from build123d import *

# Parameters (mm, degrees)
SKETCH1_W                    = 110
SKETCH1_H                    = 50
BASE_FLANGE1_DEPTH           = 6
CUT_EXTRUDE1_DEPTH           = 10
LPATTERN1_COUNT              = 2
LPATTERN1_PITCH              = 57
MIRROR1_COPY_1_DEPTH         = 10
EDGE_FLANGE1_STRIP_W         = 40
EDGE_FLANGE1_STRIP_H         = 6
EDGE_FLANGE1_STRIP_CUT_DEPTH = 50
EDGE_FLANGE1_DEPTH           = 50
EDGE_FLANGE2_STRIP_W         = 40
EDGE_FLANGE2_STRIP_H         = 6
EDGE_FLANGE2_STRIP_CUT_DEPTH = 50
EDGE_FLANGE2_DEPTH           = 50
SKETCH9_R                    = 4.5
CUT_EXTRUDE2_DEPTH           = 10


# Sheet-metal steps are written as plain solids
with BuildPart() as part:
    # Sketch1 → Base-Flange1 (new body)
    with BuildSketch(Plane(origin=(0, 0, 0), x_dir=(0, 0, -1), z_dir=(1, 0, 0))):
        Rectangle(SKETCH1_W, SKETCH1_H)
    extrude(amount=-BASE_FLANGE1_DEPTH)

    # Sketch5 → Cut-Extrude1 (cut)
    with BuildSketch(Plane.ZY.offset(6)):
        with BuildLine():
            Line((-30, 13), (-10, 13))
            ThreePointArc((-10, 13), (-7.5, 10.5), (-10, 8))
            Line((-10, 8), (-30, 8))
            ThreePointArc((-30, 8), (-32.5, 10.5), (-30, 13))
        make_face()
    cut_extrude1 = extrude(amount=-CUT_EXTRUDE1_DEPTH, mode=Mode.SUBTRACT)

    # LPattern1: Cut-Extrude1 ×2
    with Locations(*[(0, 0, i * LPATTERN1_PITCH) for i in range(1, LPATTERN1_COUNT)]):
        add(cut_extrude1, mode=Mode.SUBTRACT)

    # Mirror1: Cut-Extrude1 across plane
    add(cut_extrude1.mirror(Plane.ZX), mode=Mode.SUBTRACT)

    # Mirror1 copy 1 sketch → Mirror1 copy 1 (cut)
    with BuildSketch(Plane(origin=(-6, 0, 57), x_dir=(0, 0, 1), z_dir=(-1, 0, 0))):
        with BuildLine():
            Line((-30, -13), (-10, -13))
            ThreePointArc((-10, -13), (-7.5, -10.5), (-10, -8))
            Line((-10, -8), (-30, -8))
            ThreePointArc((-30, -8), (-32.5, -10.5), (-30, -13))
        make_face()
    extrude(amount=-MIRROR1_COPY_1_DEPTH, mode=Mode.SUBTRACT)

    # Edge-Flange1 strip (across the edge) → Edge-Flange1 strip cut (cut)
    with BuildSketch(Plane(origin=(0, -25, -55), x_dir=(0, 0, 1), z_dir=(0, 1, 0))):
        with Locations((-6, -3)):
            Rectangle(EDGE_FLANGE1_STRIP_W, EDGE_FLANGE1_STRIP_H)
    extrude(amount=EDGE_FLANGE1_STRIP_CUT_DEPTH, mode=Mode.SUBTRACT)

    # Edge-Flange1 section (across the edge) → Edge-Flange1 (add)
    with BuildSketch(Plane(origin=(0, -25, -55), x_dir=(0, 0, 1), z_dir=(0, 1, 0))):
        with BuildLine():
            Line((0, 8), (0, 67))
            Line((0, 67), (6, 67))
            Line((6, 67), (6, 8))
            ThreePointArc((6, 8), (8.343145751, 2.343145751), (14, 0))
            Line((14, 0), (14, -6))
            ThreePointArc((14, -6), (4.100505063, -1.899494937), (0, 8))
        make_face()
    extrude(amount=EDGE_FLANGE1_DEPTH)

    # Edge-Flange2 strip (across the edge) → Edge-Flange2 strip cut (cut)
    with BuildSketch(Plane(origin=(67, 25, -55), x_dir=(-1, 0, 0), z_dir=(0, -1, 0))):
        with Locations((-6, -3)):
            Rectangle(EDGE_FLANGE2_STRIP_W, EDGE_FLANGE2_STRIP_H)
    extrude(amount=EDGE_FLANGE2_STRIP_CUT_DEPTH, mode=Mode.SUBTRACT)

    # Edge-Flange2 section (across the edge) → Edge-Flange2 (add)
    with BuildSketch(Plane(origin=(67, 25, -55), x_dir=(-1, 0, 0), z_dir=(0, -1, 0))):
        with BuildLine():
            Line((0, 8), (0, 104))
            Line((0, 104), (6, 104))
            Line((6, 104), (6, 8))
            ThreePointArc((6, 8), (8.343145751, 2.343145751), (14, 0))
            Line((14, 0), (14, -6))
            ThreePointArc((14, -6), (4.100505063, -1.899494937), (0, 8))
        make_face()
    extrude(amount=EDGE_FLANGE2_DEPTH)

    # Sketch9 → Cut-Extrude2 (cut)
    with BuildSketch(Plane.ZY.offset(-61)):
        with Locations((-94, 0)):
            Circle(SKETCH9_R)
    extrude(amount=-CUT_EXTRUDE2_DEPTH, mode=Mode.SUBTRACT)

    # Mirror2: part across plane


with BuildPart() as part_1:
    add(part.part)
    add(part.part.mirror(Plane(origin=(67, 25, -159), x_dir=(1, 0, 0), z_dir=(0, 0, 1))))


solid = part_1.part
Model file for the job. Use its own axes, mm. A direction names the side the tool comes from. Give positions to 0.01 mm unless a question says otherwise; leave off trailing zeros. Order: outer loops, then holes, each group sorted by start corner. A loop starts at its lowest first (then second) coordinate and runs counter-clockwise, first axis right, second up. Notation, with made-up numbers: (-29.5, -2.75) - (-18.5, -2.75) arc R31 cw to (-18.5, 35.25) - close; hole circle Ø10 at (20.25, 11). An arc over 180 degrees is marked (long way). Return JSON: item names as keys, results as strings.
1) Cut at C-C, the plane z = -0.5. Give the cut face in (x, y), plus the area to 3 significant figures.
Geometry says:
{"outline": "(-6, -25) - (0, -25) - (0, 25) - (-6, 25) - close", "area": "300 mm²"}
2) Cut at B-B, the plane z = -94. Give the cut face in (x, y), plus the area to 3 significant figures.
Geometry says:
{"outline": "(61, -25) - (67, -25) - (67, -4.5) - (61, -4.5) - close; (61, 4.5) - (67, 4.5) - (67, 25) - (61, 25) - close", "area": "246 mm²"}
3) Cut at A-A, the plane x = 23.5. Give the cut face in (y, z), plus the area to 3 significant figures.
Geometry says:
{"outline": "(-25, -269) - (25, -269) - (25, -263) - (-25, -263) - close; (-25, -55) - (25, -55) - (25, -49) - (-25, -49) - close", "area": "600 mm²"}
4) Probe line 1 (Z direction, x = 51.5, y = -21); line 2 (Y direction, x = 63, z = -94); line 3 (X direction, y = -15, z = -185). List the from-to ranges inside material, lowest first. Write a range as from..to.
Geometry says:
{"line 1": "-269..-263, -55..-49", "line 2": "-25..-4.5, 4.5..25", "line 3": "61..67"}
5) Flat gauge pins, fed straight in: P1, Ø25, axis at y = -3, z = -332, coming from the +X side; P2, Ø4, axis at x = 36, y = 2.5, coming from the -Z side; P3, Ø8, axis at y = 0, z = -224, coming from the +X side; P4, Ø2, axis at x = 31.5, y = -8.5, coming from the +Z side. Where does each tip first touch, or does it go through?
Geometry says:
{"P1": "x = 0", "P2": "z = -269", "P3": "through", "P4": "z = -49"}
6) Pull direction Y, two halves, no side cores. Call faces 1 (the cylindrical face through (63.958, 0.198, -98.496)), 2 (the flat face through (63, -25, -190)), 3 (the flat face through (0, 0, -326)): pulls with the +Y half, pulls with the -Y half, needs draft (parallel to the pull), parting line crosses it, or undercut.
Geometry says:
{"face 1": "undercut", "face 2": "pulls with the -Y half", "face 3": "needs draft"}
7) 3-axis set-ups, long thin cutter, end or side, ignore diameter. For faces 4 (the flat face through (31, 0, -269)), 5 (the flat face through (-6, 0, 8)), 6 (the flat face through (67, 0, -160)), 7 (the flat face through (0, 0, 8)), 8 (the flat face through (30, 0, -263)): which of +Z, -Z, +X, -X, +Y, -Y reach the whole face in a straight line?
Geometry says:
{"face 4": "-Z, +X, +Y, -Y", "face 5": "+Z, -Z, -X, +Y, -Y", "face 6": "+Z, -Z, +X, +Y, -Y", "face 7": "+Z, +X, +Y, -Y", "face 8": "-X, +Y, -Y"}
